For this review, take the finished solid that the model builds, in its own axes (mm). Face numbers are marked on the shaded views. A direction names the side the tool comes from. Coordinates: 2 decimals unless noted, no trailing zeros. Loops run counter-clockwise (first coordinate to the right, second up) from the corner with the lowest first, then second, coordinate; pieces in that order, holes last. Notation, with made-up numbers: M 38,71.5 L 79,71.5 A24 ccw 79,109.5 Z; hole C 48.25,-8 d4. An arc over 180 degrees is marked long. Answer as a JSON object with one key per item and string values. Group by question number.
Item 1: Add section B-B (y = -2.5). State the section outline as (x, z) points (1 decimal).
Item 2: Mouldability with a two-part tool opening along Z and no side actions: class the marked faces 3, 4 and 5 as +Z half, -Z half, draft (parallel to the pull), parting line (faces both ways), or undercut.
Item 3: Tool access review of the marked faces 1 and 2: name each direction out of +Z, -Z, +X, -X, +Y, -Y from which nothing blocks a thin tool from reaching the whole face with its end or side.
Item 4: Insertion check: pin 1 (4 mm diameter, centred on y = 4.5, z = -5.5, fed in from +X); pin 2 (3 mm diameter, centred on y = 2, z = -11, fed in from -X); pin 3 (12 mm diameter, centred on x = -6, z = -11.5, fed in from -Y). Each pin has a flat end and moves straight along its axis. Give the tip position at first contact, or say it passes through.
Item 5: Add section C-C (y = 1.25). State the section outline as (x, z) points, then the cut area to 3 significant figures.
Item 6: Wall thickness on L1, parallel to Z at x = 0, y = -4.55; L2, parallel to Z at x = 1.75, y = -4; L3, parallel to Y at x = 0.5, z = -5.25: over which ranges is each line inside the solid? List them lowest first. Write a range as from..to.
Item 7: Add section A-A (y = -5). State the section outline as (x, z) points, then the cut area to 3 significant figures.
from build123d import *
from build123d import SkipClean  # not in build123d's __all__

# Parameters (mm, degrees)
F2_R     = 5
F2_R_2   = 3
F3_DEPTH = 0.5
F2_R_3   = 12
F4_DEPTH = 2
F5_DEPTH = 25


with BuildPart() as f1:
    # F0 (on Top) → F1 (revolve)
    with BuildSketch(Plane.XY):
        with BuildLine():
            Line((0, -5.5), (0, 0))
            Line((0, 0), (-13.25, 0))
            ThreePointArc((-13.25, 0), (-13.7144660941, -1.8708286934), (-15, -3.3071891388))
            Line((-15, -3.3071891388), (-15, -5.5))
            Line((-15, -5.5), (0, -5.5))
        make_face()
    revolve(axis=Axis((0, -2.75, 0), (0, -1, 0)))

    # F2 (on face) → F3 (join)
    with BuildSketch(Plane.XZ.offset(5.5)):
        Circle(F2_R)
        Circle(F2_R_2, mode=Mode.SUBTRACT)
    extrude(amount=F3_DEPTH)

    # F2 (on face) → F4 (cut)
    with BuildSketch(Plane.XZ.offset(5.5)):
        Circle(F2_R_3)
        Circle(F2_R, mode=Mode.SUBTRACT)
    extrude(amount=-F4_DEPTH, mode=Mode.SUBTRACT)

    # F5 (cut): a face of the model
    f5_faces = [f1.faces().sort_by_distance(p)[0] for p in [
        (0, -5.5, 0),
    ]]
    extrude(f5_faces, amount=-F5_DEPTH, mode=Mode.SUBTRACT)

    # F6: F1 across plane


with BuildPart() as f1_1:
    add(f1.part, clean=False)
    with SkipClean():  # cleaning this boolean's faces spoils the solid; the shape is the same uncleaned
        add(f1.part.mirror(Plane.XZ), clean=False)


solid = f1_1.part
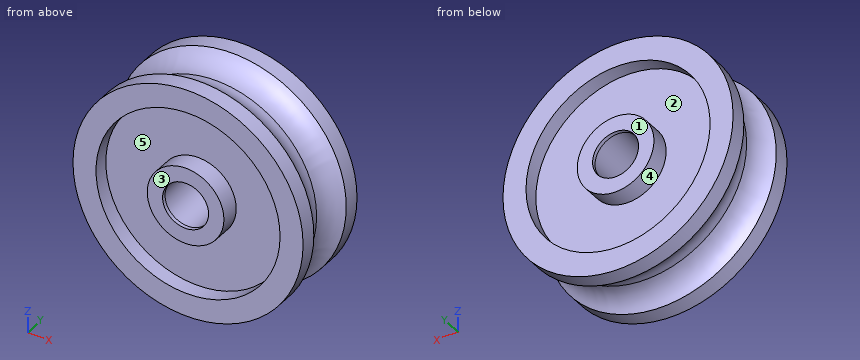
From the geometry:
{
 "1": {"outline": "C 0,0 d28.3; hole C 0,0 d6"},
 "2": {"face 3": "draft", "face 4": "undercut", "face 5": "undercut"},
 "3": {"face 1": "+Z, -Z, +X, -X, +Y", "face 2": "+Y"},
 "4": {"pin 1": "stops at x = 14.59", "pin 2": "stops at x = -10.94", "pin 3": "stops at y = -5.5"},
 "5": {"outline": "C 0,0 d26.9; hole C 0,0 d6", "area": "540 mm²"},
 "6": {"L1": "z = -15..-12, -5..-3, 3..5, 12..15", "L2": "z = -14.9..-11.87, -4.68..-2.44, 2.44..4.68, 11.87..14.9", "L3": "y = -3.5..3.5"},
 "7": {"outline": "C 0,0 d30; C 0,0 d10; hole C 0,0 d24; hole C 0,0 d6", "area": "305 mm²"}
}
